For this review, take the finished solid that the model builds, in its own axes (mm). Face numbers are marked on the shaded views. A direction names the side the tool comes from. Round coordinates to 2 decimals unless told otherwise and drop trailing zeros. Loops run counter-clockwise (first coordinate to the right, second up) from the corner with the lowest first, then second, coordinate; pieces in that order, holes last.
1. Tool access review of the marked faces 1, 2, 3 and 4: name each direction out of +Z, -Z, +X, -X, +Y, -Y from which nothing blocks a thin tool from reaching the whole face with its end or side.
2. To check wall thickness, follow line 1 along X through (y, z) = (259, 0); line 2 along Z through (x, y) = (0, -228). State the ranges of each line that lie inside material, in increasing order.
3. Consider section A-A on x = 0. State the section outline as (y, z) points, then the cut area to 3 significant figures.
4. Consider section D-D on z = -31. State the section outline as (x, y) points, then the cut area to 3 significant figures.
5. Clearance check with flat-ended pins moving along their axes: pin 1 Ø1 at (x, z) = (-97, -11.5) entering from -Y; pin 2 Ø10 at (x, z) = (49.5, -81.5) entering from +Y; pin 3 Ø2 at (x, y) = (-28, -60.5) entering from +Z; pin 4 Ø8 at (y, z) = (-103, 26.5) entering from -X. State where each tip first meets the part, or that it passes through.
6. Consider section B-B on z = 0. State the section outline as (x, y) points, then the cut area to 3 significant figures.
7. Consider section C-C on y = 192. State the section outline as (x, z) points, then the cut area to 3 significant figures.
8. Draft analysis for pull direction Z (two halves, no side actions). For the marked faces 5, 6 and 7, state which applies: released by +Z, released by -Z, zero draft, split by the parting line, or undercut.
from build123d import *

# Parameters (mm, degrees)
SKETCH1_R           = 16
BOSS_EXTRUDE1_DEPTH = 229.5
SKETCH2_R           = 52.5
BOSS_EXTRUDE2_DEPTH = 60
SKETCH3_R           = 42.5
CUT_EXTRUDE1_DEPTH  = 50
SKETCH6_R           = 50
BOSS_EXTRUDE4_DEPTH = 3.5
BOSS_EXTRUDE5_DEPTH = 240
SKETCH8_R           = 110
CUT_EXTRUDE3_DEPTH  = 50


with BuildPart() as part:
    # Sketch1 → Boss-Extrude1 (new body)
    with BuildSketch(Plane(origin=(0, 0, 0), x_dir=(1, 0, 0), z_dir=(0, 1, 0))):
        Circle(SKETCH1_R)
    extrude(amount=BOSS_EXTRUDE1_DEPTH)

    # Sketch2 → Boss-Extrude2 (add)
    with BuildSketch(Plane(origin=(0, 229.5, 0), x_dir=(1, 0, 0), z_dir=(0, 1, 0))):
        Circle(SKETCH2_R)
    extrude(amount=BOSS_EXTRUDE2_DEPTH)

    # Sketch3 → Cut-Extrude1 (cut)
    with BuildSketch(Plane(origin=(0, 289.5, 0), x_dir=(1, 0, 0), z_dir=(0, 1, 0))):
        Circle(SKETCH3_R)
    extrude(amount=-CUT_EXTRUDE1_DEPTH, mode=Mode.SUBTRACT)

    # Sketch6 → Boss-Extrude4 (add)
    with BuildSketch(Plane.XZ):
        Circle(SKETCH6_R)
    extrude(amount=BOSS_EXTRUDE4_DEPTH)

    # Sketch7 → Boss-Extrude5 (add)
    with BuildSketch(Plane.XZ.offset(3.5)):
        with BuildLine():
            Line((-126.279721603, -25), (-112.249721603, -25))
            ThreePointArc((-112.249721603, -25), (115, 0), (-112.249721603, 25))
            Line((-112.249721603, 25), (-126.279721603, 25))
            Line((-126.279721603, 25), (-126.279721603, -25))
        make_face()
    extrude(amount=BOSS_EXTRUDE5_DEPTH)

    # Sketch8 → Cut-Extrude3 (cut)
    with BuildSketch(Plane.XZ.offset(243.5)):
        Circle(SKETCH8_R)
    extrude(amount=-CUT_EXTRUDE3_DEPTH, mode=Mode.SUBTRACT)


solid = part.part
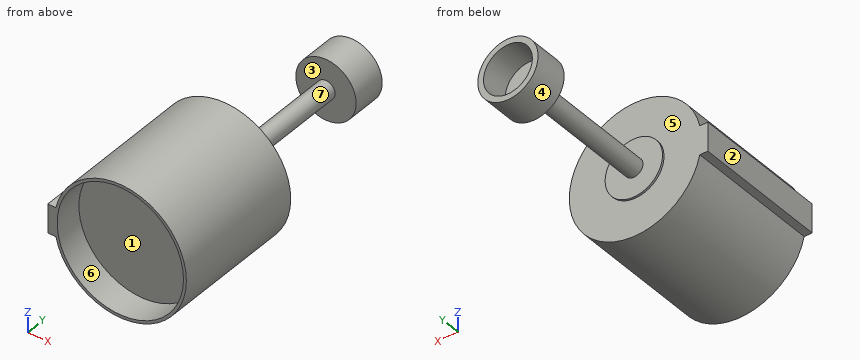
Resolved:
1. face 1: -Y
1. face 2: +Z, -Z, -X, +Y, -Y
1. face 3: none
1. face 4: +Y
2. line 1: x = -52.5 to -42.5, 42.5 to 52.5
2. line 2: z = -115 to -110, 110 to 115
3. outline: (-243.5, -115) - (-3.5, -115) - (-3.5, -50) - (0, -50) - (0, -16) - (229.5, -16) - (229.5, -52.5) - (289.5, -52.5) - (289.5, -42.5) - (239.5, -42.5) - (239.5, 42.5) - (289.5, 42.5) - (289.5, 52.5) - (229.5, 52.5) - (229.5, 16) - (0, 16) - (0, 50) - (-3.5, 50) - (-3.5, 115) - (-243.5, 115) - (-243.5, 110) - (-193.5, 110) - (-193.5, -110) - (-243.5, -110) - close
3. area: 53,900 mm2
4. outline: (-110.74, -243.5) - (-105.54, -243.5) - (-105.54, -193.5) - (105.54, -193.5) - (105.54, -243.5) - (110.74, -243.5) - (110.74, -3.5) - (39.23, -3.5) - (39.23, 0) - (-39.23, 0) - (-39.23, -3.5) - (-110.74, -3.5) - close; (-42.37, 229.5) - (42.37, 229.5) - (42.37, 289.5) - (29.07, 289.5) - (29.07, 239.5) - (-29.07, 239.5) - (-29.07, 289.5) - (-42.37, 289.5) - close
4. area: 45,100 mm2
5. pin 1: stops at y = -193.5
5. pin 2: stops at y = -3.5
5. pin 3: stops at z = 111.79
5. pin 4: stops at x = -126.28
6. outline: (-126.28, -243.5) - (-110, -243.5) - (-110, -193.5) - (110, -193.5) - (110, -243.5) - (115, -243.5) - (115, -3.5) - (50, -3.5) - (50, 0) - (16, 0) - (16, 229.5) - (52.5, 229.5) - (52.5, 289.5) - (42.5, 289.5) - (42.5, 239.5) - (-42.5, 239.5) - (-42.5, 289.5) - (-52.5, 289.5) - (-52.5, 229.5) - (-16, 229.5) - (-16, 0) - (-50, 0) - (-50, -3.5) - (-126.28, -3.5) - close
6. area: 56,700 mm2
7. outline: circle Ø32 at (0, 0)
7. area: 804 mm2
8. face 5: zero draft
8. face 6: undercut
8. face 7: split by the parting line
